```python
from build123d import *

# Parameters (mm, degrees)
F0_R      = 17.884061545
F1_DEPTH  = 1
F2_R      = 17.884061545
F2_R_2    = 15.884061545
F3_DEPTH  = 120
F5_DEPTH  = 100
F6_R      = 2
F7_DEPTH  = 121.0010007
F8_W      = 25
F8_H      = 3
F9_DEPTH  = 5
F10_R     = 1.6
F11_DEPTH = 2.5
F12_R     = 1
F13_DEPTH = 5


# Not quite as in the source:
# - a pattern or mirror of a feature is missing from the dataset's text; its kind, count and spacing are read off the source's solid
# - a feature names something its author has since deleted; it is built from what else it names


with BuildPart() as f1:
    # F0 (on Top) → F1 (new body)
    with BuildSketch(Plane.XY):
        Circle(F0_R)
    extrude(amount=F1_DEPTH)

    # F2 (on face) → F3 (join)
    with BuildSketch(Plane(origin=(0, 0, 0), x_dir=(1, 0, 0), z_dir=(0, 0, -1))):
        Circle(F2_R)
        Circle(F2_R_2, mode=Mode.SUBTRACT)
    extrude(amount=F3_DEPTH)

    # F4 (on Right) → F5 (cut, symmetric)
    with BuildSketch(Plane.YZ):
        with BuildLine():
            add(Edge.make_bspline(
                [(-23.545185104, -2.931100782), (-12.2797633222, -3.5261581086), (11.4767752963, -34.9586093489), (12.414609837, -94.1865478451), (15.1815395802, -125.3380775452)],
                knots=[0, 0, 0, 0, 0.3949910862, 1, 1, 1, 1], degree=3))
            Line((-23.545185104, -2.931100782), (-23.545185104, -130.5240243673))
            Line((-23.545185104, -130.5240243673), (15.1815395802, -125.3380775452))
        make_face()
    extrude(amount=F5_DEPTH, both=True, mode=Mode.SUBTRACT)

    # F6 (on face) → F7 (cut, through all)
    with BuildSketch(Plane.XY.offset(1)):
        with Locations((-6.0105, 6.0103152788)):
            Circle(F6_R)
        with Locations((6.0105, 6.0103152788)):
            Circle(F6_R)
        with Locations((6.0105, -6.0103152788)):
            Circle(F6_R)
        with Locations((-6.0105, -6.0103152788)):
            Circle(F6_R)
    extrude(amount=-F7_DEPTH, mode=Mode.SUBTRACT)

    # F8 (on Right) → F9 (join, symmetric)
    with BuildSketch(Plane.YZ):
        with BuildLine():
            Line((16.384061545, -77), (16.384061545, -63))
            add(Edge.make_bspline(
                [(16.384061545, -63), (16.384061545, -70), (-2.0563617415, -72.958536621), (-7.8631014511, -75.8217814094), (-8.615938455, -77)],
                knots=[0, 0, 0, 0, 0.622644618, 1, 1, 1, 1], degree=3))
            Line((-8.615938455, -77), (16.384061545, -77))
        make_face()
        with Locations((3.884061545, -78.5)):
            Rectangle(F8_W, F8_H)
    extrude(amount=F9_DEPTH, both=True)

    # F10 (on face) → F11 (join)
    with BuildSketch(Plane(origin=(0, 0, -80), x_dir=(1, 0, 0), z_dir=(0, 0, -1))):
        with Locations((0, -9.884061545)):
            Circle(F10_R)
    f11 = extrude(amount=F11_DEPTH)

    # F11_copies: F11 across plane
    add(f11.mirror(Plane(origin=(0, 3.634062, 0), x_dir=(0, 0, -1), z_dir=(0, -1, 0))))

    # F12 (on face) → F13 (cut)
    with BuildSketch(Plane(origin=(0, 0, -82.5), x_dir=(1, 0, 0), z_dir=(0, 0, -1))):
        with Locations((0, 2.615938455)):
            Circle(F12_R)
        with Locations((0, -9.884061545)):
            Circle(F12_R)
    extrude(amount=-F13_DEPTH, mode=Mode.SUBTRACT)


solid = f1.part
```
Geometry check sheet. Reference: the model listing, model coordinates, mm. A direction names the side the tool comes from. Coordinates: 2 decimals unless noted, no trailing zeros. Answer as a JSON object with one key per item and string values.
1. Go/stop test with flat-tipped pins: pin 1 Ø2.5 at (x, y) = (-0.5, 10) entering from -Z; pin 2 Ø3 at (x, z) = (-8, -63) entering from -Y; pin 3 Ø12 at (x, y) = (-4.5, 13.5) entering from -Z; pin 4 Ø0.6 at (x, y) = (0, 10.5) entering from -Z. Record where each tip stops, or that it passes through.
Answers below:
{"pin 1": "stops at z = -82.5", "pin 2": "stops at y = 12.73", "pin 3": "stops at z = -120", "pin 4": "stops at z = -77.5"}
2. Scan lines: L1, parallel to Y at x = 0, z = -80.3; L2, parallel to Y at x = 0, z = -79.55; L3, parallel to X at y = 11.5, z = -73. Record each from-to range of solid material in increasing order.
Answers below:
{"L1": "y = -4.22 to -3.62, -1.62 to -1.02, 8.28 to 8.88, 10.88 to 11.48, 15.88 to 17.88", "L2": "y = -8.62 to -3.62, -1.62 to 8.88, 10.88 to 17.88", "L3": "x = -13.7 to -10.96, -5 to 5, 10.96 to 13.7"}
3. Draft check along X on faces 1 (the flat face through (0, 0, 1)), 2 (the cylindrical face through (-3.88, 17.46, -45.21)), 3 (the flat face through (0, -3, -77.5)). Enter one of: released by +X, released by -X, zero draft, split by the parting line, or undercut.
Answers below:
{"face 1": "zero draft", "face 2": "split by the parting line", "face 3": "undercut"}
4. Tool access check on faces 4 (the cylindrical face through (-0.13, -3.607, -80.035)), 5 (the cylindrical face through (4.423, 4.793, 0.507)), 6 (the flat face through (0, 0, 0)), 7 (the flat face through (1, 9, -82.5)). Record the directions out of +Z, -Z, +X, -X, +Y, -Y that give a thin tool (end or side, any length) a straight path to the whole face; none if there is none.
Answers below:
{"face 4": "-Z", "face 5": "+Z", "face 6": "none", "face 7": "-Z, +X, -X, -Y"}
